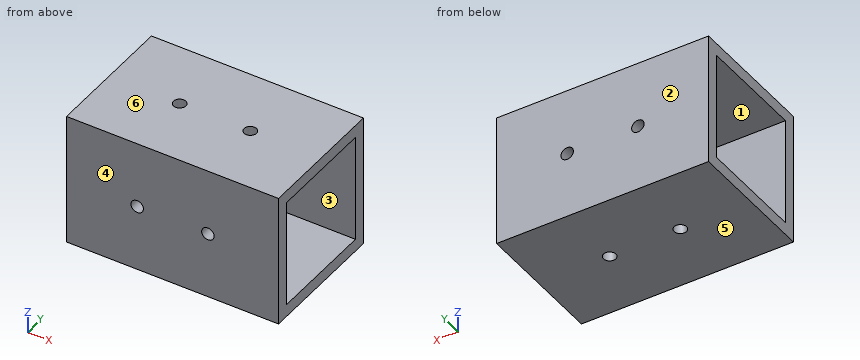
```python
from build123d import *

# Parameters (mm, degrees)
SKETCH1_W           = 50.8
SKETCH1_H           = 50.8
SKETCH1_W_2         = 41.275
SKETCH1_H_2         = 41.275
BOSS_EXTRUDE1_DEPTH = 81.025
SKETCH2_R           = 2.38125
CUT_EXTRUDE1_DEPTH  = 50.8
SKETCH3_R           = 2.38125
CUT_EXTRUDE2_DEPTH  = 52.324


with BuildPart() as part:
    # Sketch1 → Boss-Extrude1 (new body)
    with BuildSketch(Plane(origin=(0, 0, 0), x_dir=(0, 0, -1), z_dir=(1, 0, 0))):
        with Locations((-25.4, 25.4)):
            Rectangle(SKETCH1_W, SKETCH1_H)
        with Locations((-25.4, 25.4)):
            Rectangle(SKETCH1_W_2, SKETCH1_H_2, mode=Mode.SUBTRACT)
    extrude(amount=BOSS_EXTRUDE1_DEPTH)

    # Sketch2 → Cut-Extrude1 (cut)
    with BuildSketch(Plane.XY.offset(50.8)):
        with Locations((27, 25.4)):
            Circle(SKETCH2_R)
        with Locations((54.025, 25.4)):
            Circle(SKETCH2_R)
    extrude(amount=-CUT_EXTRUDE1_DEPTH, mode=Mode.SUBTRACT)

    # Sketch3 → Cut-Extrude2 (cut)
    with BuildSketch(Plane.XZ):
        with Locations((27, 25.4)):
            Circle(SKETCH3_R)
        with Locations((54.025, 25.4)):
            Circle(SKETCH3_R)
    extrude(amount=-CUT_EXTRUDE2_DEPTH, mode=Mode.SUBTRACT)


solid = part.part
```
Can you work these out from the model? Positions are in its coordinate system, mm. Face numbers are marked on the shaded views. A direction names the side the tool comes from. Give positions to 0.01 mm unless a question says otherwise; leave off trailing zeros. Loops run counter-clockwise (first coordinate to the right, second up) from the corner with the lowest first, then second, coordinate; pieces in that order, holes last. Notation, with made-up numbers: M 82,62 L 96,62 A31 ccw 96,97 Z; hole C -20.5,79.5 d11. An arc over 180 degrees is marked long. Answer in a Markdown table with one row per item.
1. Suppose I cut it at A-A on y = 17. Write out the boundary of the cut face in (x, z) (1 decimal).
Taken from the geometry:
| item | result |
|---|---|
| outline | M 0,0 L 81,0 L 81,4.8 L 0,4.8 Z; M 0,46 L 81,46 L 81,50.8 L 0,50.8 Z |
2. Suppose I cut it at B-B on z = 25.4. Write out the boundary of the cut face in (x, y) (1 decimal).
Taken from the geometry:
| item | result |
|---|---|
| outline | M 0,0 L 24.6,0 L 24.6,4.8 L 0,4.8 Z; M 0,46 L 24.6,46 L 24.6,50.8 L 0,50.8 Z; M 29.4,0 L 51.6,0 L 51.6,4.8 L 29.4,4.8 Z; M 29.4,46 L 51.6,46 L 51.6,50.8 L 29.4,50.8 Z; M 56.4,0 L 81,0 L 81,4.8 L 56.4,4.8 Z; M 56.4,46 L 81,46 L 81,50.8 L 56.4,50.8 Z |
3. Which directions (+Z, -Z, +X, -X, +Y, -Y) give clear straight access to the entire face, cutting with the end or side of a thin tool? Please do the marked faces 1 and 2.
Taken from the geometry:
| item | result |
|---|---|
| face 1 | +X, -X |
| face 2 | +Z, -Z, +X, -X, +Y |
4. If I drill on line 1 along Y through (x, z) = (51, 37); line 2 along X through (y, z) = (49, 25) (3 decimals), over which ranges is the centre line in solid material (lowest first)?
Taken from the geometry:
| item | result |
|---|---|
| line 1 | y = 0 to 4.76, 46.04 to 50.8 |
| line 2 | x = 0 to 24.653, 29.347 to 51.678, 56.372 to 81.025 |
5. For pin 1 Ø3 at (x, y) = (27, 25.4) entering from +Z, with a flat end and sliding along its axis, tell me the tip position at first contact or that it passes through.
Taken from the geometry:
| item | result |
|---|---|
| pin 1 | passes through |
6. Thinking about a two-plate mould opening in Z: for the marked faces 3, 4, 5 and 6, which applies, released by +Z, released by -Z, zero draft, split by the parting line, or undercut?
Taken from the geometry:
| item | result |
|---|---|
| face 3 | undercut |
| face 4 | zero draft |
| face 5 | released by -Z |
| face 6 | released by +Z |
